Source: CAD feature listing. Evaluate the final solid. Frame: model axes, mm. Give positions to 0.01 mm unless a question says otherwise; leave off trailing zeros. Order: outer loops, then holes, each group sorted by start corner. A loop starts at its lowest first (then second) coordinate and runs counter-clockwise, first axis right, second up. Notation, with made-up numbers: (54.25, 28) - (60.25, 28) arc R23 ccw to (60.25, 50) - close; hole circle Ø9 at (-1, 62.25). An arc over 180 degrees is marked (long way). Write each question's results on one line, items separated by ' | '. Start each with the question number.
Item 1: Contact query for a flat-ended pin moving along its axis: pin 1 Ø1.8 at (y, z) = (-19, 3) entering from -X. Output: stop coordinate, or through.
Item 2: Section B-B on x = 52.5. Output: boundary loops of the cut face in (y, z).
Item 3: Section A-A on y = 0. Output: boundary loops of the cut face in (x, z) (3 decimals), and give its area (3 significant figures).
Item 4: Section C-C on y = 21.5. State how many separate pieces and enclosed holes the cut face has, and give its area (3 significant figures).
Item 5: Line query: line 1 along Y through (x, z) = (-23, 3); line 2 along Y through (x, z) = (74, 2); line 3 along Y through (x, z) = (-20, 4.5). Output: solid intervals per line, ascending.
```python
from build123d import *

# Parameters (mm, degrees)
BOSS_EXTRUDE1_DEPTH = 6
CUT_EXTRUDE3_DEPTH  = 132.727049709
HOLE1_D             = 15
HOLE3_D             = 4.5
HOLE4_D             = 4.5


with BuildPart() as part:
    # Sketch1 → Boss-Extrude1 (new body)
    with BuildSketch(Plane(origin=(0, 0, 0), x_dir=(0, 1, 0), z_dir=(0, 0, 1))):
        Polygon((-30, 46.875), (-30, -128.125), (30, -128.125), (30, 46.875), (15, 72.855762114), (-15, 72.855762114), align=None)
    extrude(amount=BOSS_EXTRUDE1_DEPTH)

    # Sketch2 → Cut-Extrude3 (cut, through all)
    with BuildSketch(Plane.XY.offset(6)):
        Polygon((-31.286542732, 2), (-4.728430349, 2), (-18.007486541, 25), align=None)
        Polygon((106.709427996, -25), (93.430371804, -2), (106.709427996, -2), align=None)
        Polygon((-15.698085464, 25), (10.860026919, 25), (-2.419029272, 2), align=None)
        Polygon((106.709427996, 25), (106.709427996, 2), (93.430371804, 2), align=None)
        Polygon((-0.109628196, 2), (26.448484187, 2), (13.169427996, 25), align=None)
        Polygon((-46.875, 25), (-33.595943809, 2), (-20.316887617, 25), align=None)
        Polygon((15.481914536, 25), (28.760970728, 2), (42.040026919, 25), align=None)
        Polygon((44.349427996, 25), (31.070371804, 2), (57.628484187, 2), align=None)
        Polygon((46.661914536, 25), (59.940970728, 2), (73.220026919, 25), align=None)
        Polygon((75.529427996, 25), (62.250371804, 2), (88.808484187, 2), align=None)
        Polygon((77.841914536, 25), (91.120970728, 2), (104.400026919, 25), align=None)
        Polygon((77.841914536, -25), (91.120970728, -2), (104.400026919, -25), align=None)
        Polygon((75.529427996, -25), (62.250371804, -2), (88.808484187, -2), align=None)
        Polygon((46.661914536, -25), (59.940970728, -2), (73.220026919, -25), align=None)
        Polygon((44.349427996, -25), (31.070371804, -2), (57.628484187, -2), align=None)
        Polygon((15.481914536, -25), (28.760970728, -2), (42.040026919, -25), align=None)
        Polygon((13.169427996, -25), (-0.109628196, -2), (26.448484187, -2), align=None)
        Polygon((-15.698085464, -25), (-2.419029272, -2), (10.860026919, -25), align=None)
        Polygon((-18.007486541, -25), (-4.728430349, -2), (-31.286542732, -2), align=None)
        Polygon((-46.875, -25), (-33.595943809, -2), (-20.316887617, -25), align=None)
    extrude(amount=-CUT_EXTRUDE3_DEPTH, mode=Mode.SUBTRACT)

    # Hole1 (through all)
    with Locations(Plane(origin=(-54.855762114, 0, 6), x_dir=(1, 0, 0), z_dir=(0, 0, 1))):
        with Locations((0, 0)):
            Hole(HOLE1_D / 2)

    # Hole3 (through all)
    with Locations(Plane(origin=(-65.462363831, -10.606601718, 6), x_dir=(1, 0, 0), z_dir=(0, 0, 1))):
        with Locations((0, 0), (21.213203435, 0), (0, 21.213203436), (21.213203435, 21.213203436)):
            Hole(HOLE3_D / 2)

    # Hole4 (through all)
    with Locations(Plane(origin=(123.781854249, 5.656854249, 6), x_dir=(1, 0, 0), z_dir=(0, 0, 1))):
        with Locations((0, 0), (0, -11.313708498), (-11.313708498, -11.313708498), (-11.313708498, 0)):
            Hole(HOLE4_D / 2)


solid = part.part
```
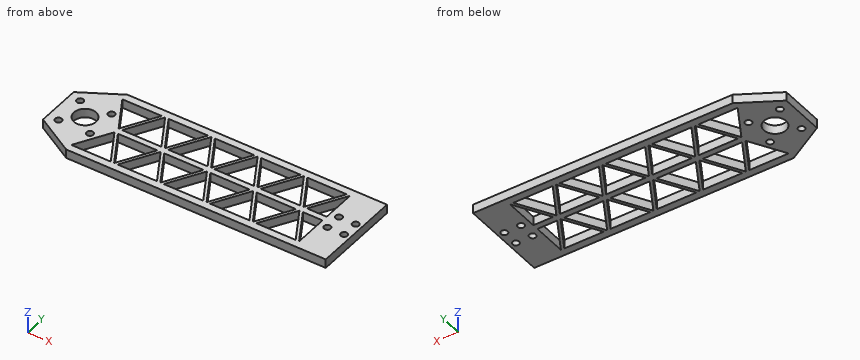
Evaluation:
1) pin 1: stops at x = -67.49
2) outline: (-30, 0) - (-25, 0) - (-25, 6) - (-30, 6) - close; (-14.89, 0) - (-10.88, 0) - (-10.88, 6) - (-14.89, 6) - close; (-2, 0) - (2, 0) - (2, 6) - (-2, 6) - close; (10.88, 0) - (14.89, 0) - (14.89, 6) - (10.88, 6) - close; (25, 0) - (30, 0) - (30, 6) - (25, 6) - close
3) outline: (-72.856, 0) - (-62.356, 0) - (-62.356, 6) - (-72.856, 6) - close; (-47.356, 0) - (128.125, 0) - (128.125, 6) - (-47.356, 6) - close | area: 1,120 mm^2
4) separate pieces: 11 | enclosed holes: 0 | area: 354 mm^2
5) line 1: y = -30 to -25, -20.35 to -16.35, -2 to 2, 16.35 to 20.35, 25 to 30 | line 2: y = -30 to -22.35, -2 to 2, 22.35 to 30 | line 3: y = -30 to -21.55, -2 to 2, 21.55 to 30
